Design review of the part built by this model. Coordinates are the model's own, in mm. Give positions to 0.01 mm unless a question says otherwise; leave off trailing zeros. Write each loop counter-clockwise with the first axis right and the second up, starting at its lowest first coordinate (ties: lowest second). Pieces come first, ordered by that corner, then holes. Notation, with made-up numbers: (6.5, -17) -> (22.5, -17) arc R18 cw to (22.5, -3) -> close; hole circle Ø8 at (-4, 78.25). An arc over 180 degrees is marked (long way). Answer as a JSON object with one key per item and string values.
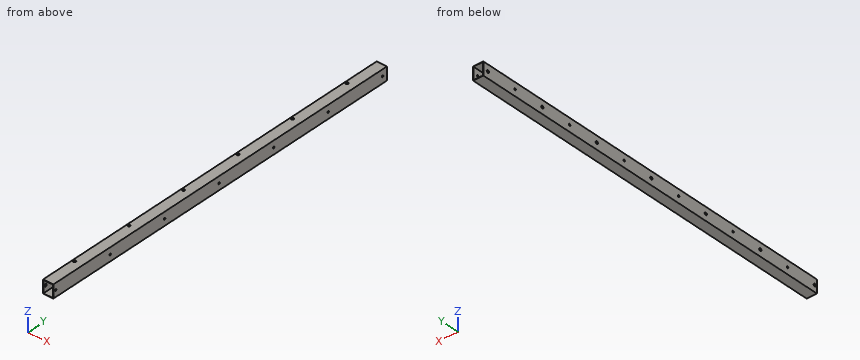
```python
from build123d import *

# Parameters (mm, degrees)
F0_W           = 40
F0_H           = 50
F0_W_2         = 37.5
F0_H_2         = 47.5
F1_DEPTH       = 1500
F4_D           = 7
F5_D           = 10
F5_DEPTH       = 20
F5_TIP         = 3.0043030951
F5_ON_F3_D     = 10
F5_ON_F3_DEPTH = 20
F5_ON_F3_TIP   = 3.0043030951
F6_D           = 7
F6_DEPTH       = 2
F6_TIP         = 2.1030121666


with BuildPart() as f1:
    # F0 (on Front) → F1 (new body)
    with BuildSketch(Plane.XZ):
        Rectangle(F0_W, F0_H)
        Rectangle(F0_W_2, F0_H_2, mode=Mode.SUBTRACT)
    extrude(amount=F1_DEPTH)

    # F4 (through all)
    with Locations(Plane(origin=(-20, 0, 0), x_dir=(0, -1, 0), z_dir=(-1, 0, 0))):
        with Locations((1490, 0), (1245, 0), (1000, 0), (755, 0), (510, 0), (265, 0), (20, 0)):
            Hole(F4_D / 2)

    # F5
    with Locations(Plane(origin=(-20, 0, 0), x_dir=(0, -1, 0), z_dir=(-1, 0, 0))):
        with Locations((1490, 0), (1245, 0), (1000, 0), (755, 0), (510, 0), (265, 0), (20, 0)):
            Hole(F5_D / 2, depth=F5_DEPTH)
            with Locations((0, 0, -(F5_DEPTH + F5_TIP / 2))):  # 118° drill point
                Cone(0, F5_D / 2, F5_TIP, mode=Mode.SUBTRACT)

    # F5 on F3
    with Locations(Plane.XY.offset(25)):
        with Locations((-12, -1367.5), (-12, -1122.5), (-12, -877.5), (-12, -632.5), (-12, -387.5), (-12, -142.5)):
            Hole(F5_ON_F3_D / 2, depth=F5_ON_F3_DEPTH)
            with Locations((0, 0, -(F5_ON_F3_DEPTH + F5_ON_F3_TIP / 2))):  # 118° drill point
                Cone(0, F5_ON_F3_D / 2, F5_ON_F3_TIP, mode=Mode.SUBTRACT)

    # F6
    with Locations(Plane(origin=(-20, 0, 0), x_dir=(0, -1, 0), z_dir=(-1, 0, 0))):
        with Locations((1367.5, 0), (1122.5, 0), (877.5, 0), (632.5, 0), (387.5, 0), (142.5, 0)):
            Hole(F6_D / 2, depth=F6_DEPTH)
            with Locations((0, 0, -(F6_DEPTH + F6_TIP / 2))):  # 118° drill point
                Cone(0, F6_D / 2, F6_TIP, mode=Mode.SUBTRACT)


solid = f1.part
```
(1) We need section A-A, the plane y = -1203. State the section outline as (x, z) points, then the cut area to 3 significant figures.
Here are the results:
{"outline": "(-20, -25) -> (20, -25) -> (20, 25) -> (-20, 25) -> close; hole (-18.75, -23.75) -> (18.75, -23.75) -> (18.75, 23.75) -> (-18.75, 23.75) -> close", "area": "219 mm²"}
(2) We need section C-C, the plane x = 1.5. State the section outline as (y, z) points.
Here are the results:
{"outline": "(-1500, -25) -> (0, -25) -> (0, -23.75) -> (-1500, -23.75) -> close; (-1500, 23.75) -> (0, 23.75) -> (0, 25) -> (-1500, 25) -> close"}
(3) We need section B-B, the plane z = -12.5. State the section outline as (x, y) points.
Here are the results:
{"outline": "(-20, -1500) -> (-18.75, -1500) -> (-18.75, 0) -> (-20, 0) -> close; (18.75, -1500) -> (20, -1500) -> (20, 0) -> (18.75, 0) -> close"}
(4) Clearance check with a flat-ended pin moving along its axis: pin 1 (9 mm diameter, centred on y = -1000, z = 0, fed in from -X). State where the tip first meets the part, or that it passes through.
Here are the results:
{"pin 1": "stops at x = 18.75"}
(5) For line 1 along X through (y, z) = (-1285.5, -15); line 2 along Z through (x, y) = (-13, -1249); line 3 along Z through (x, y) = (19.6, -510), list the stretches that pass through material, from the lowest coordinate up.
Here are the results:
{"line 1": "x = -20 to -18.75, 18.75 to 20", "line 2": "z = -25 to -23.75, 23.75 to 25", "line 3": "z = -25 to -3.5, 3.5 to 25"}
